```python
from build123d import *

# Parameters (mm, degrees)
F0_W     = 50.8
F0_H     = 50.8
F1_DEPTH = 25.4
F3_D     = 38.1
F4_R     = 3.175
F5_SIZE  = 0.635
F7_DEPTH = 50.801


with BuildPart() as f1:
    # F0 (on Top) → F1 (new body)
    with BuildSketch(Plane.XY):
        Rectangle(F0_W, F0_H)
    extrude(amount=-F1_DEPTH)

    # F3 (through all)
    with Locations(Plane.XY):
        with Locations((0, 0)):
            Hole(F3_D / 2)

    # F4
    f4_edges = [f1.edges().sort_by_distance(p)[0] for p in [
        (0, 25.4, 0),
        (25.4, 0, 0),
        (0, -25.4, 0),
        (-25.4, 0, 0),
    ]]
    fillet(f4_edges, radius=F4_R)

    # F5
    f5_edges = [f1.edges().sort_by_distance(p)[0] for p in [
        (0, 25.4, -25.4),
        (-25.4, 0, -25.4),
        (0, -25.4, -25.4),
        (25.4, 0, -25.4),
    ]]
    chamfer(f5_edges, length=F5_SIZE)

    # F6 (on face) → F7 (cut, through all)
    with BuildSketch(Plane(origin=(-25.4, 0, 0), x_dir=(0, -1, 0), z_dir=(-1, 0, 0))):
        with BuildLine():
            Line((7.355005, -16.65312), (7.355005, -8.74688))
            ThreePointArc((7.355005, -8.74688), (7.286946, -8.49288), (7.101005, -8.306939))
            Line((7.101005, -8.306939), (0.254, -4.353819))
            ThreePointArc((0.254, -4.353819), (0, -4.28576), (-0.254, -4.353819))
            Line((-0.254, -4.353819), (-7.101005, -8.306939))
            ThreePointArc((-7.101005, -8.306939), (-7.286946, -8.49288), (-7.355005, -8.74688))
            Line((-7.355005, -8.74688), (-7.355005, -16.65312))
            ThreePointArc((-7.355005, -16.65312), (-7.286946, -16.90712), (-7.101005, -17.093061))
            Line((-7.101005, -17.093061), (-0.254, -21.046181))
            ThreePointArc((-0.254, -21.046181), (0, -21.11424), (0.254, -21.046181))
            Line((0.254, -21.046181), (7.101005, -17.093061))
            ThreePointArc((7.101005, -17.093061), (7.286946, -16.90712), (7.355005, -16.65312))
        make_face()
    extrude(amount=-F7_DEPTH, mode=Mode.SUBTRACT)


solid = f1.part
```
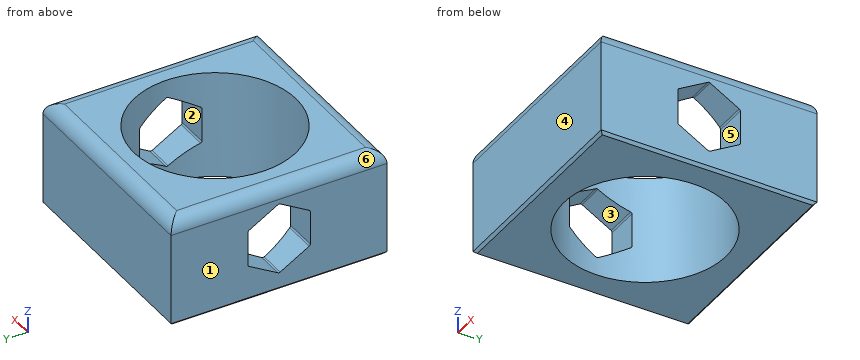
CAD build for the part. Positions are in the model's coordinates, mm. Face numbers are marked on the shaded views. A direction names the side the tool comes from. Round coordinates to 2 decimals unless told otherwise and drop trailing zeros. Loops run counter-clockwise (first coordinate to the right, second up) from the corner with the lowest first, then second, coordinate; pieces in that order, holes last. Notation, with made-up numbers: (-3, 78.5) - (46, 78.5) arc R32 cw to (46, 113.5) - close; hole circle Ø5 at (76, 23.5). An arc over 180 degrees is marked (long way). Return JSON: item names as keys, results as strings. Group by question number.
Q1. Drill centre lines: line 1 along Y through (x, z) = (0, -17.5); line 2 along Y through (x, z) = (-6, -6); line 3 along X through (y, z) = (14, -8.75). Where is each one in solid material? Low to high. Write a range as [from, to].
Q2. Band-saw the part on B-B on x = 0. Give the cut face in (y, z) (3 decimals).
Q3. Tool access for the marked faces 1 and 2: list every direction of +Z, -Z, +X, -X, +Y, -Y with a clear straight run to the whole face (end or side of a thin tool).
Q4. Two-plate mould, pull along Z, no slides. Class the marked faces 3, 4, 5 and 6: +Z half, -Z half, draft (parallel to the pull), parting line (faces both ways), or undercut.
Q5. Band-saw the part on C-C on y = 4. Give the cut face in (x, z) (3 decimals).
Q6. Band-saw the part on A-A on z = -11.75. Give the cut face in (x, y) (3 decimals), plus the area to 3 significant figures.
Solutions:
{
 "1": {"line 1": "y = [-25.4, -19.05], [19.05, 25.4]", "line 2": "y = [-25.4, -18.08], [18.08, 25.4]", "line 3": "x = [-25.4, -12.92], [12.92, 25.4]"},
 "2": {"outline": "(-25.4, -24.765) - (-24.765, -25.4) - (-19.05, -25.4) - (-19.05, 0) - (-22.225, 0) arc R3.175 ccw to (-25.4, -3.175) - close; (19.05, -25.4) - (24.765, -25.4) - (25.4, -24.765) - (25.4, -3.175) arc R3.175 ccw to (22.225, 0) - (19.05, 0) - close"},
 "3": {"face 1": "+Z, -Z, -X, +Y, -Y", "face 2": "+X, -X"},
 "4": {"face 3": "undercut", "face 4": "draft", "face 5": "undercut", "face 6": "+Z half"},
 "5": {"outline": "(-25.4, -24.765) - (-24.765, -25.4) - (-18.625, -25.4) - (-18.625, -18.883) - (-25.4, -18.883) - close; (-25.4, -6.517) - (-18.625, -6.517) - (-18.625, 0) - (-22.225, 0) arc R3.175 ccw to (-25.4, -3.175) - close; (18.625, -25.4) - (24.765, -25.4) - (25.4, -24.765) - (25.4, -18.883) - (18.625, -18.883) - close; (18.625, -6.517) - (25.4, -6.517) - (25.4, -3.175) arc R3.175 ccw to (22.225, 0) - (18.625, 0) - close"},
 "6": {"outline": "(-25.4, -25.4) - (25.4, -25.4) - (25.4, -7.355) - (17.573, -7.355) arc R19.05 cw to (-17.573, -7.355) - (-25.4, -7.355) - close; (-25.4, 7.355) - (-17.573, 7.355) arc R19.05 cw to (17.573, 7.355) - (25.4, 7.355) - (25.4, 25.4) - (-25.4, 25.4) - close", "area": "1,240 mm^2"}
}
